The model under review builds one solid part; all positions refer to its coordinate system, in mm. Face numbers are marked on the shaded views. A direction names the side the tool comes from. Round coordinates to 2 decimals unless told otherwise and drop trailing zeros. Order: outer loops, then holes, each group sorted by start corner. A loop starts at its lowest first (then second) coordinate and runs counter-clockwise, first axis right, second up. Notation, with made-up numbers: (45, -2.75) - (94, -2.75) arc R21 cw to (94, 2.25) - close; hole circle Ø5 at (88.5, 30). An arc over 180 degrees is marked (long way). One line per question, with ' | ' between items. Start each with the question number.
Item 1: For L1, parallel to Z at x = -12.5, y = 0.65; L2, parallel to X at y = 2.5, z = -8; L3, parallel to X at y = 0.95, z = 10, list the stretches that pass through material, from the lowest coordinate up. Write a range as [from, to].
Item 2: Add section C-C on x = -12.5. State the section outline as (y, z) points, and give its area (3 significant figures).
Item 3: Insertion check: pin 1 Ø3 at (x, y) = (14, 2.5) entering from -Z; pin 2 Ø2 at (x, z) = (-5.5, 6.5) entering from -Y; pin 3 Ø1 at (x, z) = (-2, -7.5) entering from +Y; pin 4 Ø1.5 at (x, z) = (-18.5, 1.5) entering from +Y. Each pin has a flat end and moves straight along its axis. Give the tip position at first contact, or say it passes through.
Item 4: Add section A-A on y = -0.75. State the section outline as (x, z) points.
Item 5: Add section B-B on z = 10. State the section outline as (x, y) points, and give its area (3 significant figures).
Item 6: Add section D-D on x = -3.5. State the section outline as (y, z) points, and give its area (3 significant figures).
Item 7: Tool access review of the marked faces 1, 2, 3, 4 and 5: name each direction out of +Z, -Z, +X, -X, +Y, -Y from which nothing blocks a thin tool from reaching the whole face with its end or side.
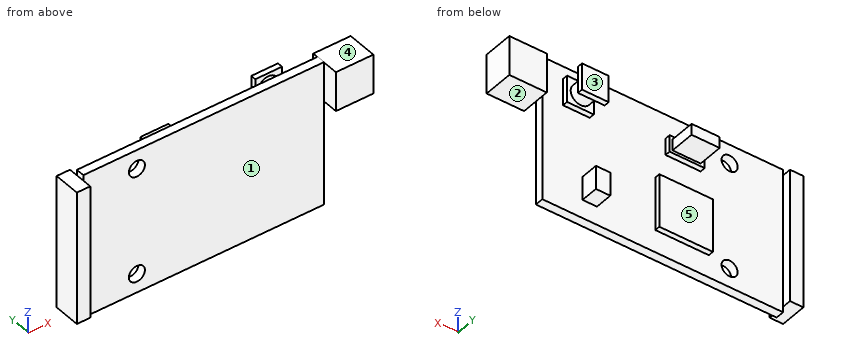
Autodesk Inventor part; units mm, degrees
ref_plane "YZ Plane" through (0, 0, 0) normal (1, 0, 0) x (0, 1, 0)
ref_plane "XZ Plane" through (0, 0, 0) normal (0, 1, 0) x (-1, 0, 0)
ref_plane "XY Plane" through (0, 0, 0) normal (0, 0, 1) x (1, 0, 0)
sketch "Boceto1" plane through (0, 0, 0) normal (0, 1, 0) x (-1, 0, 0)
  line L0 (-22.5, 13.55) -> (22.5, 13.55)
  line L1 (22.5, 13.55) -> (22.5, -13.55)
  line L2 (22.5, -13.55) -> (-22.5, -13.55)
  line L3 (-22.5, -13.55) -> (-22.5, 13.55)
  line L4 (-22.5, 13.55) -> (22.5, -13.55) construction
  line L5 (22.5, 13.55) -> (-22.5, -13.55) construction
  line L6 (22.5, 0) -> (12.5, 0)
  line L7 (12.5, 0) -> (12.5, 10)
  line L8 (12.5, 10) -> (12.5, -10)
  circle A0 centre (12.5, 10) radius 1.5
  circle A1 centre (12.5, -10) radius 1.5
  point P0 (0, 0)
  dimension "d0" = 45
  dimension "d1" = 27.1
  dimension "d2" = 10
  dimension "d3" = 10
  dimension "d4" = 20
  dimension "d5" = 3
  dimension "d6" = 3
extrude "Extrusión1" add sketch "Boceto1" along normal blind 1.6
sketch "Boceto2" plane through (-22.5, 0, -13.55) normal (-1, 0, 0) x (0, 0, 1)
  line L0 (13.55, 0) -> (13.55, 1.6)
  line L1 (27.1, 1.6) -> (0, 1.6)
  line L2 (26.05, -1.7) -> (1.05, -1.7)
  line L3 (1.05, -1.7) -> (1.05, 3.3)
  line L4 (1.05, 3.3) -> (26.05, 3.3)
  line L5 (26.05, 3.3) -> (26.05, -1.7)
  line L6 (26.05, -1.7) -> (1.05, 3.3) construction
  line L7 (1.05, -1.7) -> (26.05, 3.3) construction
  point P0 (13.55, 0.8)
  dimension "d9" = 25
  dimension "d10" = 5
extrude "Extrusión2" add sketch "Boceto2" along normal blind 2.5
sketch "Boceto3" plane through (22.5, 0, 13.55) normal (1, 0, 0) x (0, 0, -1)
  line L0 (0, 2.7012) -> (7.5, 2.7012)
  line L1 (7.5, 2.7012) -> (7.5, -2.8988)
  line L2 (7.5, -2.8988) -> (0, -2.8988)
  line L3 (0, -2.8988) -> (0, 2.7012)
  point P0 (13.55, 0)
  dimension "d13" = 7.5
  dimension "d14" = 5.6
extrude "Extrusión3" add sketch "Boceto3" along normal blind 7
sketch "Boceto4" plane through (0, 1.6, 0) normal (0, 1, 0) x (1, 0, 0)
  line L0 (-8.6118, -0.6728) -> (1.3882, -0.6728)
  line L1 (1.3882, -0.6728) -> (1.3882, 9.3272)
  line L2 (1.3882, 9.3272) -> (-8.6118, 9.3272)
  line L3 (-8.6118, 9.3272) -> (-8.6118, -0.6728)
  line L4 (-7.0868, -9.0155) -> (-0.5382, -9.0155)
  line L5 (-0.5382, -9.0155) -> (-0.5382, -5.8757)
  line L6 (-0.5382, -5.8757) -> (-7.0868, -5.8757)
  line L7 (-7.0868, -5.8757) -> (-7.0868, -9.0155)
  line L8 (12.2897, 5.6963) -> (14.9809, 5.6963)
  line L9 (14.9809, 5.6963) -> (14.9809, 10.0919)
  line L10 (14.9809, 10.0919) -> (12.2897, 10.0919)
  line L11 (12.2897, 10.0919) -> (12.2897, 5.6963)
  line L12 (13.6353, -11.1684) -> (18.6353, -11.1684)
  line L13 (18.6353, -11.1684) -> (18.6353, -6.1684)
  line L14 (18.6353, -6.1684) -> (13.6353, -6.1684)
  line L15 (13.6353, -6.1684) -> (13.6353, -11.1684)
  point P0 (0, 0)
  dimension "d17" = 10
  dimension "d18" = 10
  dimension "d19" = 5
  dimension "d20" = 5
extrude "Extrusión4" add sketch "Boceto4" along normal blind 1
sketch "Boceto5" plane through (0, 2.6, 0) normal (0, 1, 0) x (1, 0, 0)
  line L0 (-6.3329, -8.4587) -> (-1.0802, -8.4587)
  line L1 (-1.0802, -8.4587) -> (-1.0802, -6.3765)
  line L2 (-1.0802, -6.3765) -> (-6.3329, -6.3765)
  line L3 (-6.3329, -6.3765) -> (-6.3329, -8.4587)
  point P0 (0, 0)
extrude "Extrusión5" add sketch "Boceto5" along normal blind 4.7
sketch "Boceto6" plane through (0, 2.6, 0) normal (0, 1, 0) x (1, 0, 0)
  circle A0 centre (16.0574, -8.6684) radius 1.8966
  point P0 (0, 0)
extrude "Extrusión6" add sketch "Boceto6" along normal blind 2.7
sketch "Boceto7" plane through (16.0574, 5.3, 8.6684) normal (0, 1, 0) x (1, 0, 0)
  circle A0 centre (0, 0) radius 1.8966
  line L0 (2.5779, -2.5) -> (2.5779, 2.5)
  line L1 (2.5779, 2.5) -> (-2.4221, 2.5)
  line L2 (-2.4221, 2.5) -> (-2.4221, -2.5)
  line L3 (-2.4221, -2.5) -> (2.5779, -2.5)
  circle A1 centre (0, 0) radius 1.8966
  point P0 (-16.0574, 8.6684)
extrude "Extrusión7" add sketch "Boceto7" along normal blind 1 contours A0 | L3 L2 L1 L0
sketch "Boceto8" plane through (0, 2.6, 0) normal (0, 1, 0) x (1, 0, 0)
  line L0 (14.9809, 5.6963) -> (14.9809, 10.0919)
  line L1 (14.9809, 10.0919) -> (12.2897, 10.0919)
  line L2 (12.2897, 10.0919) -> (12.2897, 5.6963)
  line L3 (12.2897, 5.6963) -> (14.9809, 5.6963)
  point P0 (0, 0)
extrude "Extrusión8" add sketch "Boceto8" along normal blind 2.3
sketch "Boceto9" plane through (-22.5, 0, 13.55) normal (0, 0, 1) x (1, 0, 0)
  line L0 (52, -2.8988) -> (52, 2.7012)
  line L1 (45, -2.8988) -> (52, -2.8988)
  line L2 (52, 2.7012) -> (45, 2.7012)
  line L3 (45, 2.7012) -> (45, -2.8988)
  line L4 (45, -2.8988) -> (52, -2.8988)
  line L5 (52, -2.8988) -> (52, 2.7012)
  point P0 (22.5, 0)
extrude "Extrusión9" cut sketch "Boceto9" against normal blind 0.1
properties part number "Nano-modem"
Determined:
1) L1: [-13.55, -11.5], [-8.5, 8.5], [11.5, 13.55] | L2: [-25, -22.5], [-8.61, 1.39], [12.29, 14.98] | L3: [-25, -14], [-11, 29.5]
2) outline: (0, -13.55) - (1.6, -13.55) - (1.6, -11.5) - (0, -11.5) - close; (0, -8.5) - (1.6, -8.5) - (1.6, 8.5) - (0, 8.5) - close; (0, 11.5) - (1.6, 11.5) - (1.6, 13.55) - (0, 13.55) - close | area: 33.8 mm2
3) pin 1: z = -13.55 | pin 2: y = 0 | pin 3: y = 2.6 | pin 4: y = 1.6
4) outline: (-25, -12.5) - (-22.5, -12.5) - (-22.5, 12.5) - (-25, 12.5) - close; (22.5, 6.05) - (29.5, 6.05) - (29.5, 13.45) - (22.5, 13.45) - close
5) outline: (-25, -1.7) - (-22.5, -1.7) - (-22.5, 0) - (-14, 0) - (-14, 1.6) - (-22.5, 1.6) - (-22.5, 3.3) - (-25, 3.3) - close; (-11, 0) - (22.5, 0) - (22.5, -2.9) - (29.5, -2.9) - (29.5, 2.7) - (22.5, 2.7) - (22.5, 1.6) - (18.64, 1.6) - (18.64, 2.6) - (17.41, 2.6) - (17.41, 5.3) - (18.64, 5.3) - (18.64, 6.3) - (13.64, 6.3) - (13.64, 5.3) - (14.71, 5.3) - (14.71, 2.6) - (13.64, 2.6) - (13.64, 1.6) - (-11, 1.6) - close | area: 136 mm2
6) outline: (0, -13.55) - (1.6, -13.55) - (1.6, -9.33) - (2.6, -9.33) - (2.6, 0.67) - (1.6, 0.67) - (1.6, 5.88) - (2.6, 5.88) - (2.6, 6.38) - (7.3, 6.38) - (7.3, 8.46) - (2.6, 8.46) - (2.6, 9.02) - (1.6, 9.02) - (1.6, 13.55) - (0, 13.55) - close | area: 66.3 mm2
7) face 1: +Z, -Z, -Y | face 2: -Z, +X, +Y, -Y | face 3: +Z, -Z, +X, +Y | face 4: +Z, +X, +Y, -Y | face 5: -Z, +Y
